from build123d import *

# Parameters (mm, degrees)
CROQUIS_ZOCALO_R                   = 13
ZOCALO_DEPTH                       = 30
CROQUIS_ZOCALO_HUECO_R             = 8.2
ZOCALO_HUECO_DEPTH                 = 27
CROQUIS_BARRA_W                    = 16
CROQUIS_BARRA_H                    = 155
BARRA_DEPTH                        = 10
CROQUIS_HORQUILLA_W                = 16
CROQUIS_HORQUILLA_H                = 16
HORQUILLA_DEPTH                    = 18
HORQUILLA_RANURA_DEPTH             = 173.13366899
HORQUILLA_RANURA_DEPTH_BACK        = 173.13366899
CROQUIS_HORQUILLA_RANURA_W         = 6.4
CROQUIS_HORQUILLA_RANURA_H         = 20
EJE_CAMARA_Y_PRISIONERO_DEPTH      = 173.13366899
EJE_CAMARA_Y_PRISIONERO_DEPTH_BACK = 173.13366899
CROQUIS_EJES_R                     = 2.2
CROQUIS_EJES_R_2                   = 1.65


with BuildPart() as part:
    # Croquis_zocalo → Zocalo (new body)
    with BuildSketch(Plane(origin=(0, 0, 0), x_dir=(1, 0, 0), z_dir=(0, 1, 0))):
        with Locations(Location((0, 0, 0), (0, 0, 270))):
            Circle(CROQUIS_ZOCALO_R)
    extrude(amount=ZOCALO_DEPTH)

    # Croquis_zocalo_hueco → Zocalo_hueco (cut)
    with BuildSketch(Plane(origin=(0, 0, 0), x_dir=(1, 0, 0), z_dir=(0, 1, 0))):
        with Locations(Location((0, 0, 0), (0, 0, 270))):
            Circle(CROQUIS_ZOCALO_HUECO_R)
    extrude(amount=ZOCALO_HUECO_DEPTH, mode=Mode.SUBTRACT)

    # Croquis_barra → Barra (add)
    with BuildSketch(Plane(origin=(0, 20, 0), x_dir=(1, 0, 0), z_dir=(0, 1, 0))):
        with Locations((0, -77.5)):
            Rectangle(CROQUIS_BARRA_W, CROQUIS_BARRA_H)
    extrude(amount=BARRA_DEPTH)

    # Croquis_horquilla → Horquilla (add)
    with BuildSketch(Plane(origin=(0, 12, 0), x_dir=(1, 0, 0), z_dir=(0, 1, 0))):
        with Locations((0, -161)):
            Rectangle(CROQUIS_HORQUILLA_W, CROQUIS_HORQUILLA_H)
    extrude(amount=HORQUILLA_DEPTH)

    # Croquis_horquilla_ranura → Horquilla_ranura (cut, two sides: drawn at the far end of the back side and taken through both)
    with BuildSketch(Plane(origin=(0, 0, 0), x_dir=(1, 0, 0), z_dir=(0, 1, 0)).offset(-HORQUILLA_RANURA_DEPTH_BACK)):
        with Locations((0, -161)):
            Rectangle(CROQUIS_HORQUILLA_RANURA_W, CROQUIS_HORQUILLA_RANURA_H)
    extrude(amount=HORQUILLA_RANURA_DEPTH + HORQUILLA_RANURA_DEPTH_BACK, mode=Mode.SUBTRACT)

    # Croquis_ejes → Eje_camara_y_prisionero (cut, two sides: drawn at the far end of the back side and taken through both)
    with BuildSketch(Plane(origin=(0, 0, 0), x_dir=(0, 0, -1), z_dir=(1, 0, 0)).offset(-EJE_CAMARA_Y_PRISIONERO_DEPTH_BACK)):
        with Locations((-161, 21)):
            Circle(CROQUIS_EJES_R)
        with Locations(Location((0, 10, 0), (0, 0, 180))):
            Circle(CROQUIS_EJES_R_2)
    extrude(amount=EJE_CAMARA_Y_PRISIONERO_DEPTH + EJE_CAMARA_Y_PRISIONERO_DEPTH_BACK, mode=Mode.SUBTRACT)


solid = part.part
Geometry: final body of the model. Coordinates: model frame, mm. A direction names the side the tool comes from. Give positions to 0.01 mm unless a question says otherwise; leave off trailing zeros. Write each loop counter-clockwise with the first axis right and the second up, starting at its lowest first coordinate (ties: lowest second). Pieces come first, ordered by that corner, then holes.
(1) Mould query, pull axis Y, two halves, no side actions, for faces 5 (the cylindrical face through (10.5, 11.6, -0.4)), 6 (the flat face through (0, 20, 81)), 7 (the flat face through (0, 23, 0)), 8 (the flat face through (0, 30, 57)). Classes: released by +Y, released by -Y, zero draft, split by the parting line, or undercut.
(2) Cut plane B-B, the plane y = 10. Return loops of the section in (x, z).
(3) Cut plane A-A, the plane z = 161. Return loops of the section in (x, y).
(4) Cut plane D-D, the plane z = 78.5. Return loops of the section in (x, y).
(5) Access query for faces 1 (the flat face through (-8, 25, 91)), 2 (the flat face through (-6, 16, 153)), 3 (the flat face through (0, 20, 3)), 4 (the flat face through (3.2, 21, 158)). Directions: +Z, -Z, +X, -X, +Y, -Y. A direction counts if a zero-diameter tool reaches every point of the face in a straight line with its end or side. Return the directions, or none.
(6) First-contact query: P1, Ø14.5, axis at y = 21, z = 156, coming from the +X side; P2, Ø3, axis at x = 7.5, y = 23.5, coming from the -Z side; P3, Ø5, axis at x = 0, z = 134.5, coming from the -Y side. Flat tips, straight axial feed; report the tip coordinate or a pass-through.
(7) Ray query, line 1 (Z direction, x = 5.5, y = 21.5); line 2 (Y direction, x = -11.9, z = 0); line 3 (Z direction, x = -4.95, y = 21). Return the intervals inside material, ascending.
(8) Cut plane C-C, the plane x = 0. Return loops of the section in (y, z).
Values follow:
1. face 5: undercut
1. face 6: released by -Y
1. face 7: zero draft
1. face 8: released by +Y
2. outline: (-12.89, -1.65) arc R13 ccw to (12.89, -1.65) - (8.03, -1.65) arc R8.2 cw to (-8.03, -1.65) - close; (-12.89, 1.65) - (-8.03, 1.65) arc R8.2 cw to (8.03, 1.65) - (12.89, 1.65) arc R13 ccw to start
3. outline: (-8, 12) - (-3.2, 12) - (-3.2, 18.8) - (-8, 18.8) - close; (-8, 23.2) - (-3.2, 23.2) - (-3.2, 30) - (-8, 30) - close; (3.2, 12) - (8, 12) - (8, 18.8) - (3.2, 18.8) - close; (3.2, 23.2) - (8, 23.2) - (8, 30) - (3.2, 30) - close
4. outline: (-8, 20) - (8, 20) - (8, 30) - (-8, 30) - close
5. face 1: +Z, -X, +Y, -Y
5. face 2: +X, -X, -Y
5. face 3: -Y
5. face 4: +Z, +Y, -Y
6. P1: stops at x = 8
6. P2: stops at z = -11.53
6. P3: stops at y = 20
7. line 1: z = -11.78 to -6.08, 0 to 158.86, 163.14 to 169
7. line 2: y = 0 to 8.35, 11.65 to 30
7. line 3: z = -12.02 to -6.54, 0 to 158.8, 163.2 to 169
8. outline: (0, -13) - (30, -13) - (30, 151) - (20, 151) - (20, 13) - (0, 13) - (0, 8.2) - (20, 8.2) - (20, 0) - (27, 0) - (27, -8.2) - (0, -8.2) - close
